Source: three-view drawing plus pictorial views. Frame: mm from the lowest corner of the part. A direction names the side the tool comes from. Round coordinates to 2 decimals unless told otherwise and drop trailing zeros. Order: outer loops, then holes, each group sorted by start corner. A loop starts at its lowest first (then second) coordinate and runs counter-clockwise, first axis right, second up. Notation, with made-up numbers: M -40,85.5 L -30,85.5 A29 ccw -30,114.5 Z; hole C 53,62 d8. An arc over 180 degrees is marked long. Return JSON: item names as keys, results as strings. Group by question number.
Q1. Contact query for flat-ended pins moving along their axis: pin 1 (1.5 mm diameter, centred on y = 34.5, z = 5, fed in from +X); pin 2 (1.8 mm diameter, centred on x = 17.5, z = 8, fed in from +Y); pin 3 (1 mm diameter, centred on x = 5.5, z = 17, fed in from +Y). Output: stop coordinate, or through.
Q2. Ray query, probe 1 along Z at (x, y) = (17.5, 21.5); probe 2 along X at (y, z) = (18.75, 17.5); probe 3 along X at (y, z) = (25, 17). Return the intervals inside material, ascending.
Q3. Access query for the marked faces 1 and 2. Directions: +Z, -Z, +X, -X, +Y, -Y. A direction counts if a zero-diameter tool reaches every point of the face in a straight line with its end or side. Return the directions, or none.
Q4. Cut plane B-B on y = 10.5. Output: boundary loops of the cut face in (x, z).
Q5. Cut plane D-D on y = 49.5. Output: boundary loops of the cut face in (x, z).
Q6. Cut plane C-C on x = 17.5. Output: boundary loops of the cut face in (y, z), and give its area (3 significant figures).
Q7. Cut plane A-A on z = 17.5. Output: boundary loops of the cut face in (x, y).
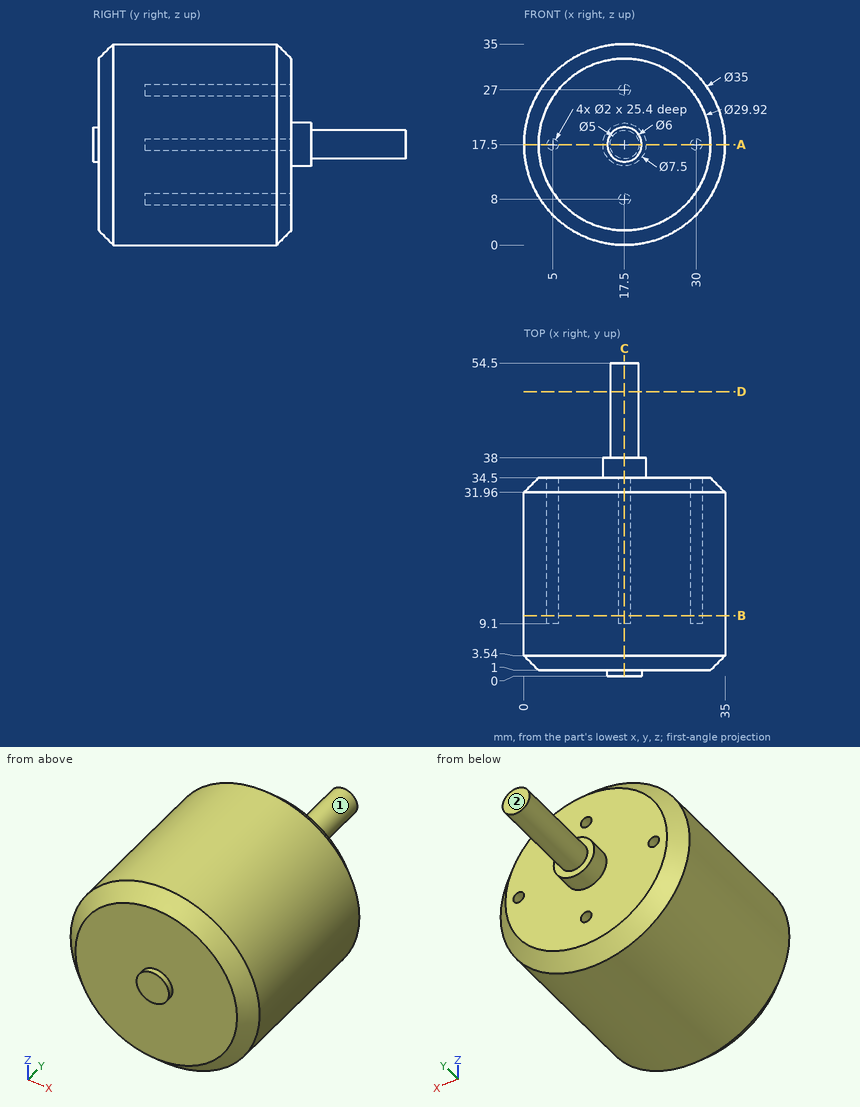
Result sheet:
{
 "1": {"pin 1": "stops at x = 27.34", "pin 2": "stops at y = 9.1", "pin 3": "stops at y = 34.5"},
 "2": {"probe 1": "z = 0 to 7, 9 to 26, 28 to 35", "probe 2": "x = 0 to 4, 6 to 29, 31 to 35", "probe 3": "x = 0.01 to 4.13, 5.87 to 29.13, 30.87 to 34.99"},
 "3": {"face 1": "+Y", "face 2": "+Z, -Z, +X, -X, +Y"},
 "4": {"outline": "C 17.5,17.5 d35; hole C 5,17.5 d2; hole C 17.5,8 d2; hole C 17.5,27 d2; hole C 30,17.5 d2"},
 "5": {"outline": "C 17.5,17.5 d5"},
 "6": {"outline": "M 0,14.5 L 1,14.5 L 1,2.54 L 3.54,0 L 31.96,0 L 34.5,2.54 L 34.5,7 L 9.1,7 L 9.1,9 L 34.5,9 L 34.5,13.75 L 38,13.75 L 38,15 L 54.5,15 L 54.5,20 L 38,20 L 38,21.25 L 34.5,21.25 L 34.5,26 L 9.1,26 L 9.1,28 L 34.5,28 L 34.5,32.46 L 31.96,35 L 3.54,35 L 1,32.46 L 1,20.5 L 0,20.5 Z", "area": "1,170 mm²"},
 "7": {"outline": "M 0,3.54 L 2.54,1 L 14.5,1 L 14.5,0 L 20.5,0 L 20.5,1 L 32.46,1 L 35,3.54 L 35,31.96 L 32.46,34.5 L 31,34.5 L 31,9.1 L 29,9.1 L 29,34.5 L 21.25,34.5 L 21.25,38 L 20,38 L 20,54.5 L 15,54.5 L 15,38 L 13.75,38 L 13.75,34.5 L 6,34.5 L 6,9.1 L 4,9.1 L 4,34.5 L 2.54,34.5 L 0,31.96 Z"}
}
